Could you check a few things on this model? Use its own coordinates, in mm. A direction names the side the tool comes from. Give positions to 0.01 mm unless a question says otherwise; leave off trailing zeros. Loops run counter-clockwise (first coordinate to the right, second up) from the corner with the lowest first, then second, coordinate; pieces in that order, holes last. Notation, with made-up numbers: (-26, 27.25) -> (-22, 27.25) arc R10 ccw to (-22, 36.25) -> close; hole circle Ø6 at (14, 20). An arc over 180 degrees is marked (long way). Put each result on its own line as item: value.
```python
from build123d import *

# Parameters (mm, degrees)
SKETCH1_W           = 11.5
SKETCH1_H           = 7.8
BOSS_EXTRUDE1_DEPTH = 223.2
SKETCH2_W           = 0.835250229
SKETCH2_H           = 1.6
CUT_EXTRUDE1_DEPTH  = 224.308111138
SKETCH3_R           = 3
CUT_EXTRUDE2_DEPTH  = 4.7
SKETCH4_R           = 1.7
CUT_EXTRUDE3_DEPTH  = 224.323515331


with BuildPart() as part:
    # Sketch1 → Boss-Extrude1 (new body)
    with BuildSketch(Plane.XY):
        Rectangle(SKETCH1_W, SKETCH1_H)
    extrude(amount=BOSS_EXTRUDE1_DEPTH)

    # Sketch2 → Cut-Extrude1 (cut, through all)
    with BuildSketch(Plane.XY.offset(223.2)):
        with Locations((5.332374886, 1.7)):
            Rectangle(SKETCH2_W, SKETCH2_H)
        with Locations((-5.332374886, 1.7)):
            Rectangle(SKETCH2_W, SKETCH2_H)
    extrude(amount=-CUT_EXTRUDE1_DEPTH, mode=Mode.SUBTRACT)

    # Sketch3 → Cut-Extrude2 (cut)
    with BuildSketch(Plane(origin=(0, 3.9, 0), x_dir=(1, 0, 0), z_dir=(0, 1, 0))):
        with Locations(Location((0, -211.6, 0), (0, 0, 270))):
            Circle(SKETCH3_R)
        with Locations(Location((0, -187.5, 0), (0, 0, 270))):
            Circle(SKETCH3_R)
        with Locations(Location((0, -163.4, 0), (0, 0, 270))):
            Circle(SKETCH3_R)
        with Locations(Location((0, -139.3, 0), (0, 0, 270))):
            Circle(SKETCH3_R)
        with Locations(Location((0, -115.2, 0), (0, 0, 270))):
            Circle(SKETCH3_R)
        with Locations(Location((0, -91.1, 0), (0, 0, 270))):
            Circle(SKETCH3_R)
        with Locations(Location((0, -67, 0), (0, 0, 270))):
            Circle(SKETCH3_R)
        with Locations(Location((0, -42.9, 0), (0, 0, 270))):
            Circle(SKETCH3_R)
        with Locations(Location((0, -18.8, 0), (0, 0, 270))):
            Circle(SKETCH3_R)
    extrude(amount=-CUT_EXTRUDE2_DEPTH, mode=Mode.SUBTRACT)

    # Sketch4 → Cut-Extrude3 (cut, through all)
    with BuildSketch(Plane(origin=(0, -0.8, 0), x_dir=(1, 0, 0), z_dir=(0, 1, 0))):
        with Locations(Location((0, -211.6, 0), (0, 0, 270))):
            Circle(SKETCH4_R)
        with Locations(Location((0, -187.5, 0), (0, 0, 270))):
            Circle(SKETCH4_R)
        with Locations(Location((0, -163.4, 0), (0, 0, 270))):
            Circle(SKETCH4_R)
        with Locations(Location((0, -139.3, 0), (0, 0, 270))):
            Circle(SKETCH4_R)
        with Locations(Location((0, -115.2, 0), (0, 0, 270))):
            Circle(SKETCH4_R)
        with Locations(Location((0, -91.1, 0), (0, 0, 270))):
            Circle(SKETCH4_R)
        with Locations(Location((0, -67, 0), (0, 0, 270))):
            Circle(SKETCH4_R)
        with Locations(Location((0, -42.9, 0), (0, 0, 270))):
            Circle(SKETCH4_R)
        with Locations(Location((0, -18.8, 0), (0, 0, 270))):
            Circle(SKETCH4_R)
    extrude(amount=-CUT_EXTRUDE3_DEPTH, mode=Mode.SUBTRACT)


solid = part.part
```
1. I need wall thicknesses on line 1 (X direction, y = -2.35, z = 139.3); line 2 (X direction, y = 2.3, z = 187.5); line 3 (Y direction, x = 2, z = 212.5). Which ranges of each line are inside material? Lowest first, please.
Recorded:
line 1: x = -5.75 to -1.7, 1.7 to 5.75
line 2: x = -4.91 to -3, 3 to 4.91
line 3: y = -3.9 to -0.8
2. If we section it at A-A (z = 56): List the corners of the cut face in (x, y) for me, then the cut area to 3 significant figures.
Recorded:
outline: (-5.75, -3.9) -> (5.75, -3.9) -> (5.75, 0.9) -> (4.91, 0.9) -> (4.91, 2.5) -> (5.75, 2.5) -> (5.75, 3.9) -> (-5.75, 3.9) -> (-5.75, 2.5) -> (-4.91, 2.5) -> (-4.91, 0.9) -> (-5.75, 0.9) -> close
area: 87.0 mm^2
3. Thinking about a two-plate mould opening in Z: for faces 3 (the face through (0, 0, 0)), 4 (the face through (0, 0, 223.2)), 5 (the face through (0, 3.9, 110)), 6 (the face through (0.1, 1.6, 15.8)), which applies, pulls with the +Z half, pulls with the -Z half, needs draft (parallel to the pull), parting line crosses it, or undercut?
Recorded:
face 3: pulls with the -Z half
face 4: pulls with the +Z half
face 5: needs draft
face 6: undercut
4. I'm going to push flat-ended pins straight in: pin 1 (3 mm diameter, centred on x = -0.5, z = 189, fed in from +Y); pin 2 (2 mm diameter, centred on x = 0, z = 115.2, fed in from +Y); pin 3 (5.5 mm diameter, centred on x = 0, z = 163.4, fed in from +Y). Where does each tip first touch, or does it pass through?
Recorded:
pin 1: stops at y = 3.9
pin 2: passes through
pin 3: stops at y = -0.8
5. For faces 1 (the face through (-1, -0.8, 141)), 2 (the face through (5.75, -2, 110)), which set-ups out of +Z, -Z, +X, -X, +Y, -Y let a thin tool reach every point of the face, with its end or its side?
Recorded:
face 1: +Y
face 2: +Z, -Z, +X, +Y, -Y
